```python
from build123d import *

# Parameters (mm, degrees)
F0_W     = 8
F0_H     = 6
F0_R     = 2.5
F1_DEPTH = 5
F3_DEPTH = 25
F0_R_2   = 2
F4_DEPTH = 5
F5_R     = 2
F6_R     = 0.25
F7_R     = 0.2


with BuildPart() as f1:
    # F0 (on Top) → F1 (new body)
    with BuildSketch(Plane.XY):
        Rectangle(F0_W, F0_H)
        Circle(F0_R, mode=Mode.SUBTRACT)
    extrude(amount=F1_DEPTH)

    # F2 (on face) → F3 (cut)
    with BuildSketch(Plane.XZ.offset(3)):
        Polygon((-4, 5), (-4, 0.2), (4, 1.210635), (4, 5), align=None)
    extrude(amount=-F3_DEPTH, mode=Mode.SUBTRACT)

    # F0 (on Top) → F4 (join)
    with BuildSketch(Plane.XY):
        Circle(F0_R)
        Circle(F0_R_2, mode=Mode.SUBTRACT)
    extrude(amount=F4_DEPTH)

    # F5
    f5_edges = [f1.edges().sort_by_distance(p)[0] for p in [
        (4, 3, 0.605318),
        (-4, 3, 0.1),
        (-4, -3, 0.1),
        (4, -3, 0.605318),
    ]]
    fillet(f5_edges, radius=F5_R)

    # F6
    f6_edges = [f1.edges().sort_by_distance(p)[0] for p in [
        (0, 3, 0),
        (3.414214, 2.414214, 0),
        (-3.414214, 2.414214, 0),
        (4, 0, 0),
        (-4, 0, 0),
        (3.414214, -2.414214, 0),
        (-3.414214, -2.414214, 0),
        (0, -3, 0),
        (-2, 0, 0),
    ]]
    fillet(f6_edges, radius=F6_R)

    # F7
    f7_edges = [f1.edges().sort_by_distance(p)[0] for p in [
        (-2, 0, 5),
        (-2.5, 0, 5),
    ]]
    fillet(f7_edges, radius=F7_R)


solid = f1.part
```
The listing builds one solid part. Answer for the finished solid, in the listing's coordinates (mm). A direction names the side the tool comes from. Round coordinates to 2 decimals unless told otherwise and drop trailing zeros. Loops run counter-clockwise (first coordinate to the right, second up) from the corner with the lowest first, then second, coordinate; pieces in that order, holes last. Notation, with made-up numbers: (54.25, 64) - (104.25, 64) arc R33 ccw to (104.25, 101) - close; hole circle Ø5 at (14.5, 0). An arc over 180 degrees is marked (long way). Return JSON: item names as keys, results as strings. Group by question number.
1. The part is cut by section A-A on x = 0. Determine the outline of the cut face in (y, z).
2. The mould has two halves that part along X. Classify faces 3 (the cylindrical face through (0, -2, 2)), 4 (the cylindrical face through (3.43, 2.4, 0.74)), 5 (the flat face through (-0.1, -2.4, 0)): pulls with the +X half, pulls with the -X half, needs draft (parallel to the pull), parting line crosses it, or undercut.
3. Each of these flat-tipped pins is pushed along its axis until it touches: P1, Ø3, axis at y = -1, z = 1, coming from the -X side; P2, Ø1, axis at x = 0, z = 2.5, coming from the +Y side; P3, Ø1.5, axis at y = 0, z = 4.5, coming from the +X side. Where does it stop, or does it pass through?
4. The part is cut by section C-C on z = 2.65. Determine the outline of the cut face in (x, y).
5. The part is cut by section B-B on z = 0.75. Determine the outline of the cut face in (x, y), then the cut area to 3 significant figures.
6. Which of the six approach directions +Z, -Z, +X, -X, +Y, -Y give full straight-line access (tool end or side, diameter ignored) to faces 1 (the flat face through (4, 0, 1)), 2 (the flat face through (-0.056, -2.709, 0.698))?
7. Consider probe 1 along Y at (x, z) = (0, 0.8); probe 2 along X at (y, z) = (1.75, 0.85); probe 3 along X at (y, z) = (-1, 2.9). Determine where each line is inside the solid, lowest interval first.
Resolved:
{
 "1": {"outline": "(-3, 0.25) arc R0.25 ccw to (-2.75, 0) - (-2.25, 0) arc R0.25 ccw to (-2, 0.25) - (-2, 4.8) arc R0.2 ccw to (-2.2, 5) - (-2.3, 5) arc R0.2 ccw to (-2.5, 4.8) - (-2.5, 0.71) - (-3, 0.71) - close; (2, 0.25) arc R0.25 ccw to (2.25, 0) - (2.75, 0) arc R0.25 ccw to (3, 0.25) - (3, 0.71) - (2.5, 0.71) - (2.5, 4.8) arc R0.2 ccw to (2.3, 5) - (2.2, 5) arc R0.2 ccw to (2, 4.8) - close"},
 "2": {"face 3": "undercut", "face 4": "pulls with the +X half", "face 5": "needs draft"},
 "3": {"P1": "stops at x = -4", "P2": "stops at y = 2.5", "P3": "stops at x = 2.5"},
 "4": {"outline": "circle Ø5 at (0, 0); hole circle Ø4 at (0, 0)"},
 "5": {"outline": "(0.35, -3) - (2, -3) arc R2 ccw to (4, -1) - (4, 1) arc R2 ccw to (2, 3) - (0.35, 3) - (0.35, 2.47) arc R2.5 ccw (long way) to (0.35, -2.47) - close; hole circle Ø4 at (0, 0)", "area": "19.2 mm²"},
 "6": {"face 1": "+Z, -Z, +X, +Y, -Y", "face 2": "+Z"},
 "7": {"probe 1": "y = -2.5 to -2, 2 to 2.5", "probe 2": "x = -1.79 to -0.97, 0.97 to 3.85", "probe 3": "x = -2.29 to -1.73, 1.73 to 2.29"}
}
